Geometry: final body of the model. Coordinates: model frame, mm. A direction names the side the tool comes from. Coordinates: 2 decimals unless noted, no trailing zeros. Loops run counter-clockwise (first coordinate to the right, second up) from the corner with the lowest first, then second, coordinate; pieces in that order, holes last. Notation, with made-up numbers: (78.25, -32.5) - (112.25, -32.5) arc R17 ccw to (112.25, -2.5) - close; hole circle Ø5 at (-25, -37). An arc over 180 degrees is marked (long way). Put each result on its own line as item: value. Start each with the question number.
1) Section D-D on x = 12. Output: boundary loops of the cut face in (y, z), and give its area (3 significant figures).
2) Contact query for flat-ended pins moving along their axis: pin 1 Ø1 at (x, y) = (3.5, 1) entering from +Z; pin 2 Ø4 at (x, z) = (-3.5, -5) entering from +Y; pin 3 Ø12 at (x, y) = (7.5, 2) entering from -Z; pin 4 Ø10 at (x, y) = (7, -1.5) entering from +Z. Output: stop coordinate, or through.
3) Material intervals for line 1 along Z through (x, y) = (0, -11); line 2 along Y through (x, z) = (0, 3); line 3 along Y through (x, z) = (-1, -6.5), sorted ascending. Write a range as from..to.
4) Section A-A on x = 0. Output: boundary loops of the cut face in (y, z).
5) Reachability of faces 1 (the flat face through (0, 0, 1)), 2 (the flat face through (0, -10.13, -1)), 3 (the flat face through (0, 14.067, 3)) from +Z, -Z, +X, -X, +Y, -Y: full face, straight path, thin tool, end or side. Return the list, or none.
6) Draft query along X for faces 4 (the cylindrical face through (-7.007, 6.426, 3.638)), 5 (the flat face through (0, 2, 0)), 6 (the flat face through (-17.678, 0, 2)). Return one class per face: +X half, -X half, draft (parallel to the pull), parting line (faces both ways), or undercut.
7) Section C-C on y = 0. Output: boundary loops of the cut face in (x, z).
8) Section B-B on z = -3.81. Output: boundary loops of the cut face in (x, y).
```python
from build123d import *

# Parameters (mm, degrees)
F0_W     = 35.35511
F0_H     = 28.1335
F0_R     = 9.5075
F1_DEPTH = 1
F2_DEPTH = 6.35
F3_W     = 35.35511
F3_H     = 7.62
F3_R     = 2.5908
F4_DEPTH = 3.937


with BuildPart() as f1:
    # F0 (on Top) → F1 (new body)
    with BuildSketch(Plane.XY):
        Rectangle(F0_W, F0_H)
        Circle(F0_R, mode=Mode.SUBTRACT)
        Circle(F0_R)
    extrude(amount=F1_DEPTH)

    # F0 (on Top) → F2 (join)
    with BuildSketch(Plane.XY):
        Rectangle(F0_W, F0_H)
        Circle(F0_R, mode=Mode.SUBTRACT)
    extrude(amount=F2_DEPTH)

    # F3 (on face) → F4 (join)
    with BuildSketch(Plane.XZ.offset(14.06675)):
        with Locations((0, -3.81)):
            Rectangle(F3_W, F3_H)
        with Locations((0, -3.81)):
            Circle(F3_R, mode=Mode.SUBTRACT)
    extrude(amount=-F4_DEPTH)


solid = f1.part
```
Answer block:
1. outline: (-14.07, -7.62) - (-10.13, -7.62) - (-10.13, 0) - (14.07, 0) - (14.07, 6.35) - (-14.07, 6.35) - close
1. area: 209 mm²
2. pin 1: stops at z = 1
2. pin 2: stops at y = -10.13
2. pin 3: stops at z = 0
2. pin 4: stops at z = 6.35
3. line 1: z = -7.62..-6.4, -1.22..6.35
3. line 2: y = -14.07..-9.51, 9.51..14.07
3. line 3: y = -14.07..-10.13
4. outline: (-14.07, -7.62) - (-10.13, -7.62) - (-10.13, -6.4) - (-14.07, -6.4) - close; (-14.07, -1.22) - (-10.13, -1.22) - (-10.13, 0) - (14.07, 0) - (14.07, 6.35) - (9.51, 6.35) - (9.51, 1) - (-9.51, 1) - (-9.51, 6.35) - (-14.07, 6.35) - close
5. face 1: +Z
5. face 2: -Z, +X, -X, +Y
5. face 3: +Z, -Z, +X, -X, +Y
6. face 4: undercut
6. face 5: draft
6. face 6: -X half
7. outline: (-17.68, 0) - (17.68, 0) - (17.68, 6.35) - (9.51, 6.35) - (9.51, 1) - (-9.51, 1) - (-9.51, 6.35) - (-17.68, 6.35) - close
8. outline: (-17.68, -14.07) - (-2.59, -14.07) - (-2.59, -10.13) - (-17.68, -10.13) - close; (2.59, -14.07) - (17.68, -14.07) - (17.68, -10.13) - (2.59, -10.13) - close
